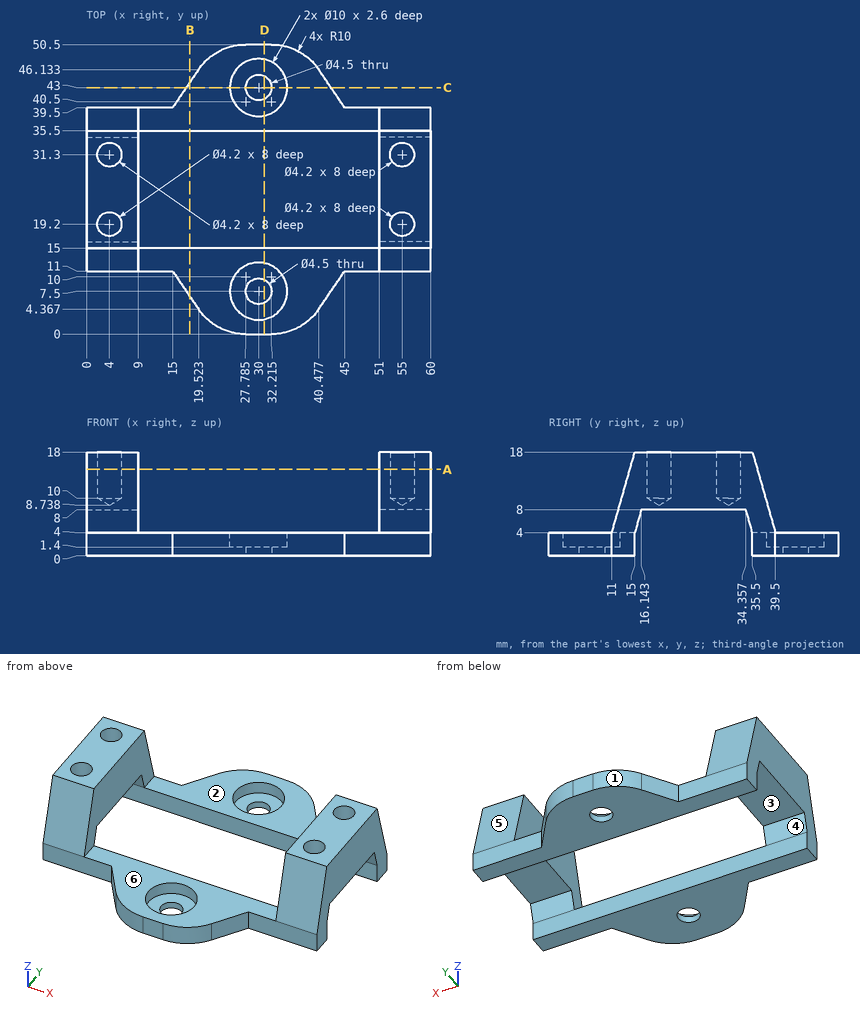
Input: dimensioned drawing with shaded views. Units: mm. Origin: part minimum x, y, z. A direction names the side the tool comes from. Give positions to 0.01 mm unless a question says otherwise; leave off trailing zeros. Write each loop counter-clockwise with the first axis right and the second up, starting at its lowest first coordinate (ties: lowest second). Pieces come first, ordered by that corner, then holes.
1. Draft query along X for the marked faces 1, 2 and 3. Return one class per face: released by +X, released by -X, zero draft, split by the parting line, or undercut.
2. Pin query (flat end, axial travel): P1, Ø6, axis at y = 10.5, z = 5.5, coming from the -X side; P2, Ø5, axis at x = 4, y = 31.3, coming from the -Z side; P3, Ø8, axis at x = 14, y = 32, coming from the +Z side; P4, Ø4.5, axis at x = 11, z = 2.5, coming from the +Y side. Return the tip coordinate at first contact, or that it passes through.
3. Section query C-C, the plane y = 43. Return loops of the section in (x, z).
4. Section query B-B, the plane x = 18. Return loops of the section in (y, z).
5. Section query A-A, the plane z = 15. Return loops of the section in (x, y).
6. Reachability of the marked faces 4, 5 and 6 from +Z, -Z, +X, -X, +Y, -Y: full face, straight path, thin tool, end or side. Return the list, or none.
7. Line query: probe 1 along Y at (x, z) = (30, 2.6); probe 2 along Y at (x, z) = (30, 0.65); probe 3 along X at (y, z) = (16, 9.5). Output: solid intervals per line, ascending.
8. Section query D-D, the plane x = 31. Return loops of the section in (y, z) (1 decimal).
Computed:
1. face 1: released by -X
1. face 2: undercut
1. face 3: zero draft
2. P1: stops at x = 0
2. P2: stops at z = 8
2. P3: stops at z = 4
2. P4: stops at y = 39.5
3. outline: (17.39, 0) - (27.75, 0) - (27.75, 1.4) - (25, 1.4) - (25, 4) - (17.39, 4) - close; (32.25, 0) - (42.61, 0) - (42.61, 4) - (35, 4) - (35, 1.4) - (32.25, 1.4) - close
4. outline: (6.6, 0) - (15, 0) - (15, 4) - (6.6, 4) - close; (35.5, 0) - (43.9, 0) - (43.9, 4) - (35.5, 4) - close
5. outline: (0, 14.14) - (9, 14.14) - (9, 36.36) - (0, 36.36) - close; (51, 14.14) - (60, 14.14) - (60, 36.36) - (51, 36.36) - close; hole circle Ø4.2 at (4, 19.2); hole circle Ø4.2 at (4, 31.3); hole circle Ø4.2 at (55, 19.2); hole circle Ø4.2 at (55, 31.3)
6. face 4: -Z, +X, -X
6. face 5: +Z, +X, -X, +Y
6. face 6: +Z, +Y, -Y
7. probe 1: y = 0 to 2.5, 12.5 to 15, 35.5 to 38, 48 to 50.5
7. probe 2: y = 0 to 5.25, 9.75 to 15, 35.5 to 40.75, 45.25 to 50.5
7. probe 3: x = 0 to 9, 51 to 60
8. outline: (0, 0) - (5.5, 0) - (5.5, 1.4) - (2.6, 1.4) - (2.6, 4) - (0, 4) - close; (9.5, 0) - (15, 0) - (15, 4) - (12.4, 4) - (12.4, 1.4) - (9.5, 1.4) - close; (35.5, 0) - (41, 0) - (41, 1.4) - (38.1, 1.4) - (38.1, 4) - (35.5, 4) - close; (45, 0) - (50.5, 0) - (50.5, 4) - (47.9, 4) - (47.9, 1.4) - (45, 1.4) - close
